```python
from build123d import *

# Parameters (mm, degrees)
SKETCH1_R           = 46.875
SKETCH1_R_2         = 12.5
BOSS_EXTRUDE1_DEPTH = 50


with BuildPart() as part:
    # Sketch1 → Boss-Extrude1 (new body)
    with BuildSketch(Plane.ZY):
        with BuildLine():
            Line((-86.671705253, -75), (-700, -75))
            ThreePointArc((-700, -75), (-775, 0), (-700, 75))
            Line((-700, 75), (0, 75))
            ThreePointArc((0, 75), (37.522455225, 64.938935577), (64.977821402, 37.455076103))
            Line((64.977821402, 37.455076103), (389.588480961, -525.686042712))
            ThreePointArc((389.588480961, -525.686042712), (362.065735663, -628.118940217), (259.632838158, -600.596194918))
            Line((259.632838158, -600.596194918), (-21.693883852, -112.544923897))
            ThreePointArc((-21.693883852, -112.544923897), (-49.149250028, -85.061064423), (-86.671705253, -75))
        make_face()
        with Locations((-700, 0)):
            Circle(SKETCH1_R, mode=Mode.SUBTRACT)
        Circle(SKETCH1_R, mode=Mode.SUBTRACT)
        with Locations((324.61065956, -563.141118815)):
            Circle(SKETCH1_R_2, mode=Mode.SUBTRACT)
    extrude(amount=BOSS_EXTRUDE1_DEPTH)


solid = part.part
```
The listing builds one solid part. Answer for the finished solid, in the listing's coordinates (mm). Coordinates: 2 decimals unless noted, no trailing zeros. Write each loop counter-clockwise with the first axis right and the second up, starting at its lowest first coordinate (ties: lowest second). Pieces come first, ordered by that corner, then holes. Notation, with made-up numbers: (28.5, -11.5) - (71.5, -11.5) arc R17 ccw to (71.5, -6.5) - close; hole circle Ø11 at (-24.5, 0.25). An arc over 180 degrees is marked (long way). One line per item, written item: value.
1) Find section C-C (z = -100.5). Give the vertices of the cut face in (x, y), and give its area (3 significant figures).
Geometry check:
outline: (-50, -75) - (0, -75) - (0, 75) - (-50, 75) - close
area: 7,500 mm2
2) For a pull along Y with two mould halves and no side action, classify faces 1 (the flat face through (-50, -69, -98)), 2 (the flat face through (-25, -75, -389)), 3 (the cylindrical face through (-24.65, 39.525, 25.2)) as pulls with the +Y half, pulls with the -Y half, needs draft (parallel to the pull), parting line crosses it, or undercut.
Geometry check:
face 1: needs draft
face 2: pulls with the -Y half
face 3: undercut
3) Each of these flat-tipped pins is pushed along its axis until it touches: pin 1 Ø1 at (x, y) = (-20, -60) entering from +Z; pin 2 Ø4 at (x, z) = (-22.5, 131) entering from -Y; pin 3 Ø2 at (x, z) = (-25.5, -463.5) entering from -Y. Where does it stop, or does it pass through?
Geometry check:
pin 1: stops at z = 121.44
pin 2: stops at y = -380.91
pin 3: stops at y = -75
4) Consider line 1 along Y through (x, z) = (-39, -700.5); line 2 along Y through (x, z) = (-4, -253.5); line 3 along Z through (x, y) = (-28, -20). Determine where each line is inside the solid, lowest interval first. Write a range as from..to.
Geometry check:
line 1: y = -75..-46.87, 46.87..75
line 2: y = -75..75
line 3: z = -772.28..-742.39, -657.61..-42.39, 42.39..98.1
5) Find section B-B (x = -21.5). Give the vertices of the cut face in (y, z) (3 decimals), and give its area (3 significant figures).
Geometry check:
outline: (-600.596, 259.633) - (-112.545, -21.694) arc R75 cw to (-75, -86.672) - (-75, -700) arc R75 ccw to (75, -700) - (75, 0) arc R75 ccw to (37.455, 64.978) - (-525.686, 389.588) arc R75 ccw to start; hole circle Ø25 at (-563.141, 324.611); hole circle Ø93.75 at (0, -700); hole circle Ø93.75 at (0, 0)
area: 206,000 mm2
6) Find section D-D (y = -204). Give the vertices of the cut face in (x, z).
Geometry check:
outline: (-50, 31.02) - (0, 31.02) - (0, 204.16) - (-50, 204.16) - close
7) Find section A-A (y = 0). Give the vertices of the cut face in (x, z) (3 decimals), and give its area (3 significant figures).
Geometry check:
outline: (-50, -775) - (0, -775) - (0, -746.875) - (-50, -746.875) - close; (-50, -653.125) - (0, -653.125) - (0, -46.875) - (-50, -46.875) - close; (-50, 46.875) - (0, 46.875) - (0, 86.568) - (-50, 86.568) - close
area: 33,700 mm2
